from build123d import *

# Parameters (mm, degrees)
SKETCH_R              = 8.8
PAD_DEPTH             = 108
SKETCH001_R           = 5.8
PAD001_DEPTH          = 5
SKETCH002_W           = 5
SKETCH002_H           = 2.6
POCKET_DEPTH          = 5
POLARPATTERN_COUNT    = 2
POCKET001_DEPTH       = 3
POLARPATTERN001_COUNT = 2
PAD002_DEPTH          = 5
POLARPATTERN002_COUNT = 2


with BuildPart() as part:
    # Sketch → Pad (new body)
    with BuildSketch(Plane.XY):
        Circle(SKETCH_R)
    extrude(amount=PAD_DEPTH)

    # Sketch001 → Pad001 (join)
    with BuildSketch(Plane.XY.offset(108)):
        Circle(SKETCH001_R)
    extrude(amount=PAD001_DEPTH)

    # Sketch002 → Pocket (cut)
    with BuildSketch(Plane.XY.offset(108)):
        with Locations((7.65, 0)):
            Rectangle(SKETCH002_W, SKETCH002_H)
    pocket = extrude(amount=POCKET_DEPTH, mode=Mode.SUBTRACT)

    # PolarPattern: Pocket ×2 about axis
    polarpattern_axis = Axis((0, 0, 108), (0, 0, 1))
    for i in range(1, POLARPATTERN_COUNT):
        add(pocket.rotate(polarpattern_axis, i * 360 / POLARPATTERN_COUNT), mode=Mode.SUBTRACT)

    # Sketch003 (on Face3 of PolarPattern) → Pocket001 (cut)
    with BuildSketch(Plane.XY.offset(108)):
        with BuildLine():
            ThreePointArc((3.6416, -3.6416), (4.75798, -1.97082), (5.15, 0))
            Line((8, 0), (5.15, 0))
            ThreePointArc((5.656854, -5.656854), (7.391036, -3.061467), (8, 0))
            Line((3.6416, -3.6416), (5.656854, -5.656854))
        make_face()
    pocket001 = extrude(amount=POCKET001_DEPTH, mode=Mode.SUBTRACT)

    # PolarPattern001: Pocket001 ×2 about axis
    polarpattern001_axis = Axis((0, 0, 108), (0, 0, 1))
    for i in range(1, POLARPATTERN001_COUNT):
        add(pocket001.rotate(polarpattern001_axis, i * 360 / POLARPATTERN001_COUNT), mode=Mode.SUBTRACT)

    # Sketch004 (on Face3 of PolarPattern001) → Pad002 (join)
    with BuildSketch(Plane.XY.offset(108)):
        with BuildLine():
            ThreePointArc((4.933386, -1.795606), (5.007014, -1.578705), (5.071111, -1.3588))
            Line((5.071111, -1.3588), (0, 0))
            Line((4.933386, -1.795606), (0, 0))
        make_face()
    pad002 = extrude(amount=PAD002_DEPTH)

    # PolarPattern002: Pad002 ×2 about axis
    polarpattern002_axis = Axis((0, 0, 108), (0, 0, 1))
    for i in range(1, POLARPATTERN002_COUNT):
        add(pad002.rotate(polarpattern002_axis, i * 360 / POLARPATTERN002_COUNT))


solid = part.part
Input: part model. Units: mm. Frame: model coordinates. A direction names the side the tool comes from. Give positions to 0.01 mm unless a question says otherwise; leave off trailing zeros. Order: outer loops, then holes, each group sorted by start corner. A loop starts at its lowest first (then second) coordinate and runs counter-clockwise, first axis right, second up. Notation, with made-up numbers: (15, 80.25) - (38, 80.25) arc R37 cw to (38, 118.25) - close; hole circle Ø1 at (35, -37). An arc over 180 degrees is marked (long way). Answer as a JSON object with one key per item and string values. Group by question number.
Q1. Set-up query: faces 1 (the face through (8.394, 2.643, 53.244)), 2 (the face through (-5.15, -0.3, 111)). Return all of +Z, -Z, +X, -X, +Y, -Y with unobstructed straight access to the full face (end or side cutting, diameter ignored); none if empty.
Q2. Mould query, pull axis Y, two halves, no side actions, for faces 3 (the face through (5.15, 0.3, 111)), 4 (the face through (0, 0, 113)), 5 (the face through (-1.81, -5.51, 110.46)), 6 (the face through (1.81, 5.51, 110.46)). Classes: pulls with the +Y half, pulls with the -Y half, needs draft (parallel to the pull), parting line crosses it, or undercut.
Q3. Cut plane A-A, the plane x = 0. Output: boundary loops of the cut face in (y, z).
Q4. Line query: probe 1 along Z at (x, y) = (3.75, 7.5); probe 2 along X at (y, z) = (-0.25, 10); probe 3 along Y at (x, z) = (-0.5, 52.5). Output: solid intervals per line, ascending.
Q5. First-contact query: pin 1 Ø3 at (y, z) = (6, 15.5) entering from +X; pin 2 Ø4 at (x, z) = (3, 39.5) entering from +Y; pin 3 Ø0.8 at (y, z) = (0.5, 110) entering from -X; pin 4 Ø4 at (x, y) = (6, 3) entering from +Z. Flat tips, straight axial feed; report the tip coordinate or a pass-through.
Q6. Cut plane B-B, the plane z = 77. Output: boundary loops of the cut face in (x, y), then the cut area to 3 significant figures.
Q7. Cut plane C-C, the plane x = 7.25. Output: boundary loops of the cut face in (y, z), then the cut area to 3 significant figures.
Results:
{
 "1": {"face 1": "+Z, -Z", "face 2": "+Z, -X"},
 "2": {"face 3": "undercut", "face 4": "needs draft", "face 5": "pulls with the -Y half", "face 6": "pulls with the +Y half"},
 "3": {"outline": "(-8.8, 0) - (8.8, 0) - (8.8, 108) - (5.8, 108) - (5.8, 113) - (-5.8, 113) - (-5.8, 108) - (-8.8, 108) - close"},
 "4": {"probe 1": "0 to 108", "probe 2": "-8.8 to 8.8", "probe 3": "-8.79 to 8.79"},
 "5": {"pin 1": "x = 7.56", "pin 2": "y = 8.74", "pin 3": "x = -5.15", "pin 4": "z = 113"},
 "6": {"outline": "circle Ø17.6 at (0, 0)", "area": "243 mm^2"},
 "7": {"outline": "(-4.99, 0) - (4.99, 0) - (4.99, 108) - (-4.99, 108) - close", "area": "1,080 mm^2"}
}
